Work out the finished part from the listing and answer in its coordinate system (mm). A direction names the side the tool comes from. Coordinates: 2 decimals unless noted, no trailing zeros. Order: outer loops, then holes, each group sorted by start corner. A loop starts at its lowest first (then second) coordinate and runs counter-clockwise, first axis right, second up. Notation, with made-up numbers: (-12, 45) - (8, 45) arc R18 cw to (8, 72) - close; hole circle Ø9 at (24.25, -25). An arc over 180 degrees is marked (long way). Answer as a JSON object with one key per item and string values. Group by question number.
1) The mould has two halves that part along Y. Classify faces 4 (the face through (1, -6, 0)), 5 (the face through (0, 3, -1)), 6 (the face through (3.23, 0.27, -9.22)), 7 (the face through (10.07, -3.275, 3.349)): released by +Y, released by -Y, zero draft, split by the parting line, or undercut.
2) A tool of negligible diameter and unlimited length cuts with its end or side. For faces 1 (the face through (3.23, -6.75, 0.05)), 2 (the face through (10.07, 4.09, -4.39)), 3 (the face through (1.5, -5, 5)), from which of +Z, -Z, +X, -X, +Y, -Y can it reach the whole face along a straight path? Write none if from no direction.
3) Find the intervals of material crossed by line 1 along X through (y, z) = (5.75, 8.5); line 2 along Z through (x, y) = (4.35, 8); line 3 along Y through (x, z) = (13.25, 1.75), in increasing order.
4) Section B-B (z = -8.5) is taken. Give the vertices of the cut face in (x, y).
5) Section A-A (y = 0) is taken. Give the vertices of the cut face in (x, z).
6) Each of these flat-tipped pins is pushed along its axis until it touches: P1, Ø1.5, axis at y = -8, z = 0, coming from the +X side; P2, Ø1, axis at y = 2.5, z = -8, coming from the +X side; P3, Ø1, axis at x = 12.5, y = -2, coming from the -Z side; P4, Ø5, axis at x = 13.5, z = 5, coming from the -Y side. Where does it stop, or does it pass through?
7) Section C-C (y = -8) is taken. Give the vertices of the cut face in (x, z), plus the area to 3 significant figures.
8) Section D-D (x = 10.25) is taken. Give the vertices of the cut face in (y, z), plus the area to 3 significant figures.
from build123d import *

# Parameters (mm, degrees)
SKETCH001_R     = 1.25
POCKET_DEPTH    = 5
POCKET001_DEPTH = 5
POCKET002_DEPTH = 10


with BuildPart() as part:
    # Sketch → Revolution (revolve)
    with BuildSketch(Plane.XY):
        Polygon((0, 3), (0, 6), (1.5, 6), (1.5, 11), (5, 11), (5, 6), (15, 6), (15, 3), align=None)
    revolve(axis=Axis((0, 0, 0), (1, 0, 0)))

    # Sketch001 (on Face3 of Revolution) → Pocket (cut)
    with BuildSketch(Plane(origin=(1.5, 0, 0), x_dir=(0, -1, 0), z_dir=(-1, 0, 0))):
        with Locations((0, 8)):
            Circle(SKETCH001_R)
        with Locations((-8, 0)):
            Circle(SKETCH001_R)
        with Locations((8, 0)):
            Circle(SKETCH001_R)
        with Locations((0, -8)):
            Circle(SKETCH001_R)
    extrude(amount=-POCKET_DEPTH, mode=Mode.SUBTRACT)

    # Sketch004 (on Face5 of Pocket) → Pocket001 (cut)
    with BuildSketch(Plane(origin=(1.5, 0, 0), x_dir=(0, -1, 0), z_dir=(-1, 0, 0))):
        with BuildLine():
            Line((-10.993204, -0.386602), (-0.386602, -10.993204))
            ThreePointArc((-10.993204, -0.386602), (-7.778175, -7.778175), (-0.386602, -10.993204))
        make_face()
    extrude(amount=-POCKET001_DEPTH, mode=Mode.SUBTRACT)

    # Sketch005 (on Face4 of Pocket001) → Pocket002 (cut)
    with BuildSketch(Plane.YZ.offset(15)):
        with BuildLine():
            Line((-0.66026, 5.963561), (-5.963561, 0.66026))
            ThreePointArc((-0.66026, 5.963561), (-4.242641, 4.242641), (-5.963561, 0.66026))
        make_face()
    extrude(amount=-POCKET002_DEPTH, mode=Mode.SUBTRACT)


solid = part.part
Report:
{
 "1": {"face 4": "split by the parting line", "face 5": "zero draft", "face 6": "undercut", "face 7": "released by -Y"},
 "2": {"face 1": "+X, -X", "face 2": "+X", "face 3": "-X"},
 "3": {"line 1": "x = 1.5 to 5", "line 2": "z = -3.38 to -1.25, 1.25 to 7.55", "line 3": "y = -4.87 to -2.44, 2.44 to 5.74"},
 "4": {"outline": "(1.5, -6.98) - (5, -6.98) - (5, -1.15) - (1.5, -1.15) - close; (1.5, 1.15) - (5, 1.15) - (5, 2.88) - (1.5, 2.88) - close"},
 "5": {"outline": "(0, -6) - (1.5, -6) - (1.5, -6.75) - (5, -6.75) - (5, -6) - (15, -6) - (15, -3) - (0, -3) - close; (0, 3) - (15, 3) - (15, 6) - (5, 6) - (5, 6.75) - (1.5, 6.75) - (1.5, 6) - (0, 6) - close; (1.5, -11) - (5, -11) - (5, -9.25) - (1.5, -9.25) - close; (1.5, 9.25) - (5, 9.25) - (5, 11) - (1.5, 11) - close"},
 "6": {"P1": "passes through", "P2": "stops at x = 5", "P3": "stops at z = -5.81", "P4": "stops at y = -4.12"},
 "7": {"outline": "(1.5, -7.55) - (5, -7.55) - (5, -1.25) - (1.5, -1.25) - close; (1.5, 1.25) - (5, 1.25) - (5, 7.55) - (1.5, 7.55) - close", "area": "44.1 mm²"},
 "8": {"outline": "(-5.96, 0.66) arc R6 ccw (long way) to (-0.66, 5.96) - close; hole circle Ø6 at (0, 0)", "area": "78.1 mm²"}
}
